CAD build for the part. Positions are in the model's coordinates, mm. A direction names the side the tool comes from. Round coordinates to 2 decimals unless told otherwise and drop trailing zeros. Loops run counter-clockwise (first coordinate to the right, second up) from the corner with the lowest first, then second, coordinate; pieces in that order, holes last. Notation, with made-up numbers: (-9.5, -26) -> (44.5, -26) arc R15 cw to (44.5, -13) -> close; hole circle Ø8 at (68.25, 4). An arc over 180 degrees is marked (long way). Answer as CSV lines item,"result".
```python
from build123d import *

# Parameters (mm, degrees)
F0_W     = 15
F0_H     = 25
F1_DEPTH = 4
F2_W     = 5
F2_H     = 25
F3_DEPTH = 14
F4_R     = 3.5
F4_R_2   = 1.725
F5_DEPTH = 2
F6_DEPTH = 4
F7_R     = 1.725
F8_DEPTH = 5
F9_R     = 4
F10_R    = 2.49999


# Not quite as in the source:
# - a fillet or chamfer is up to 0.001 mm smaller than in the source, because OpenCascade refuses the exact size


with BuildPart() as f1:
    # F0 (on Top) → F1 (new body)
    with BuildSketch(Plane.XY):
        with Locations((7.5, 12.5)):
            Rectangle(F0_W, F0_H)
    extrude(amount=F1_DEPTH)

    # F2 (on face) → F3 (join)
    with BuildSketch(Plane.XY.offset(4)):
        with Locations((2.5, 12.5)):
            Rectangle(F2_W, F2_H)
    extrude(amount=F3_DEPTH)

    # F4 (on face) → F5 (cut)
    with BuildSketch(Plane.XY.offset(4)):
        with Locations((10, 19)):
            Circle(F4_R)
        with Locations((10, 19)):
            Circle(F4_R_2, mode=Mode.SUBTRACT)
        with Locations((10, 6)):
            Circle(F4_R)
        with Locations((10, 6)):
            Circle(F4_R_2, mode=Mode.SUBTRACT)
    extrude(amount=-F5_DEPTH, mode=Mode.SUBTRACT)

    # F4 (on face) → F6 (cut, through all)
    with BuildSketch(Plane.XY.offset(4)):
        with Locations((10, 19)):
            Circle(F4_R_2)
        with Locations((10, 6)):
            Circle(F4_R_2)
    extrude(amount=-F6_DEPTH, mode=Mode.SUBTRACT)

    # F7 (on face) → F8 (cut, through all)
    with BuildSketch(Plane.YZ.offset(5)):
        with Locations((7.75, 11)):
            Circle(F7_R)
        with Locations((17.25, 11)):
            Circle(F7_R)
    extrude(amount=-F8_DEPTH, mode=Mode.SUBTRACT)

    # F9
    f9_edges = [f1.edges().sort_by_distance(p)[0] for p in [
        (15, 0, 2),
        (15, 25, 2),
    ]]
    fillet(f9_edges, radius=F9_R)

    # F10 (radius 2.5 in the source; OpenCascade refuses exactly that, so slightly less here)
    f10_edges = [f1.edges().sort_by_distance(p)[0] for p in [
        (0, 0, 9),
        (0, 25, 9),
        (5, 25, 11),
        (5, 0, 11),
    ]]
    fillet(f10_edges, radius=F10_R)


solid = f1.part
```
Q1. Drop flat-ended pins along their axis: pin 1 Ø1 at (y, z) = (18, 9) entering from +X; pin 2 Ø9 at (x, y) = (10, 6) entering from -Z; pin 3 Ø5 at (x, y) = (8, 19.5) entering from +Z; pin 4 Ø4 at (x, y) = (10, 19) entering from +Z. Give the stop position or say it passes through.
Results:
pin 1,"x = 5"
pin 2,"z = 0"
pin 3,"z = 4"
pin 4,"z = 2"
Q2. Probe L1, parallel to Y at x = 10, z = 1.2 (3 decimals); L2, parallel to Y at x = 10, z = 3.5; L3, parallel to Z at x = 13, y = 4.75. List the from-to ranges inside material, lowest first. Write a range as [from, to].
Results:
L1,"[0, 4.275], [7.725, 17.275], [20.725, 25]"
L2,"[0, 2.5], [9.5, 15.5], [22.5, 25]"
L3,"[0, 2]"
Q3. Two-plate mould, pull along Y, no slides. Class faces 1 (the cylindrical face through (7.2, 3.9, 3)), 2 (the flat face through (10, 13, 4)), 3 (the cylindrical face through (0.713, 24.248, 8.874)): pulls with the +Y half, pulls with the -Y half, needs draft (parallel to the pull), parting line crosses it, or undercut.
Results:
face 1,"undercut"
face 2,"needs draft"
face 3,"pulls with the +Y half"
Q4. Tool access for faces 4 (the cylindrical face through (4.287, 24.248, 11.098)), 5 (the flat face through (5, 12, 11)), 6 (the flat face through (11, 21, 2)), 7 (the cylindrical face through (4.248, 0.713, 11.098)): list every direction of +Z, -Z, +X, -X, +Y, -Y with a clear straight run to the whole face (end or side of a thin tool).
Results:
face 4,"+Z, +X, +Y"
face 5,"+Z, +X, +Y, -Y"
face 6,"+Z"
face 7,"+Z, +X, -Y"
Q5. Slice it at D-D, the plane y = 14. Give the cut face in (x, z), and give its area (3 significant figures).
Results:
outline,"(0, 0) -> (15, 0) -> (15, 4) -> (5, 4) -> (5, 18) -> (0, 18) -> close"
area,"130 mm2"
Q6. Slice it at B-B, the plane y = 19.5. Give the cut face in (x, z), and give its area (3 significant figures).
Results:
outline,"(0, 0) -> (8.35, 0) -> (8.35, 2) -> (6.54, 2) -> (6.54, 4) -> (5, 4) -> (5, 18) -> (0, 18) -> close; (11.65, 0) -> (15, 0) -> (15, 4) -> (13.46, 4) -> (13.46, 2) -> (11.65, 2) -> close"
area,"110 mm2"
Q7. Slice it at A-A, the plane z = 11. Count the separate pieces of the cut face and the enclosed holes in it, and give its area (3 significant figures).
Results:
separate pieces,"3"
enclosed holes,"0"
area,"85.1 mm2"
